Geometry: final body of the model. Coordinates: model frame, mm. Face numbers are marked on the shaded views. A direction names the side the tool comes from. Give positions to 0.01 mm unless a question says otherwise; leave off trailing zeros. Write each loop counter-clockwise with the first axis right and the second up, starting at its lowest first coordinate (ties: lowest second). Pieces come first, ordered by that corner, then holes. Notation, with made-up numbers: (25.25, -38) -> (30.25, -38) arc R18 ccw to (30.25, -22) -> close; hole circle Ø3 at (-39, -0.5). An arc over 180 degrees is marked (long way). Answer as a JSON object with one key per item and string values. Group by question number.
(1) Draft query along Y for the marked faces 4, 5 and 6. Return one class per face: +Y half, -Y half, draft (parallel to the pull), parting line (faces both ways), or undercut.
(2) Section query A-A on y = 15.5. Output: boundary loops of the cut face in (x, z), plus the area to 3 significant figures.
(3) Set-up query: the marked faces 1, 2 and 3. Return all of +Z, -Z, +X, -X, +Y, -Y with unobstructed straight access to the full face (end or side cutting, diameter ignored); none if empty.
(4) Contact query for flat-ended pins moving along their axis: pin 1 Ø12 at (y, z) = (25, 4) entering from +X; pin 2 Ø17 at (y, z) = (-0.5, -4.5) entering from +X; pin 3 Ø2 at (x, z) = (5.5, 12) entering from +Y; pin 4 Ø5 at (x, y) = (9.5, 3.5) entering from -Z. Output: stop coordinate, or through.
(5) Material intervals for probe 1 along Y at (x, z) = (4.25, 0); probe 2 along Y at (x, z) = (8.75, 0); probe 3 along X at (y, z) = (20.5, 13), sorted ascending.
(6) Section query C-C on y = -1. Output: boundary loops of the cut face in (x, z), plus the area to 3 significant figures.
(7) Section query B-B on x = 9. Output: boundary loops of the cut face in (y, z).
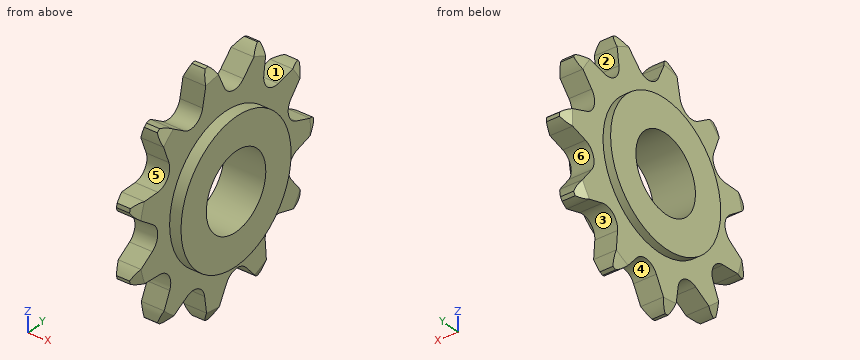
from build123d import *

# Parameters (mm, degrees)
SKETCH1_R           = 18.5
SKETCH1_R_2         = 10
BOSS_EXTRUDE1_DEPTH = 11
BOSS_EXTRUDE2_START = -6
SKETCH2_R           = 31.5
SKETCH2_R_2         = 10
BOSS_EXTRUDE2_DEPTH = 6
CHAMFER1_SIZE       = 1.27
CHAMFER1_SIZE2      = 2.723523789
CUT_EXTRUDE1_DEPTH  = 46.885727629
CIRPATTERN1_COUNT   = 11


with BuildPart() as part:
    # Sketch1 → Boss-Extrude1 (new body)
    with BuildSketch(Plane(origin=(0, 0, 0), x_dir=(0, 0, -1), z_dir=(1, 0, 0))):
        Circle(SKETCH1_R)
        Circle(SKETCH1_R_2, mode=Mode.SUBTRACT)
    extrude(amount=BOSS_EXTRUDE1_DEPTH)

    # Sketch2 → Boss-Extrude2 (add)
    with BuildSketch(Plane(origin=(7.999999904, 0, 0), x_dir=(0, 0, -1), z_dir=(1, 0, 0)).offset(BOSS_EXTRUDE2_START)):
        Circle(SKETCH2_R)
        Circle(SKETCH2_R_2, mode=Mode.SUBTRACT)
    extrude(amount=BOSS_EXTRUDE2_DEPTH)

    # Chamfer1
    chamfer1_edges = [part.edges().sort_by_distance(p)[0] for p in [
        (7.999999904, 0, 31.5),
        (1.999999904, 0, 31.5),
    ]]
    chamfer1_side = [part.faces().sort_by_distance(p)[0] for p in [
        (4.999999904, 0, 31.5),
    ]]
    chamfer(chamfer1_edges, length=CHAMFER1_SIZE, length2=CHAMFER1_SIZE2, reference=chamfer1_side[0])

    # Sketch3 → Cut-Extrude1 (cut, through all)
    with BuildSketch(Plane(origin=(11, 0, 0), x_dir=(0, 0, -1), z_dir=(1, 0, 0))):
        with BuildLine():
            Line((2.025004531, 28.705137864), (3.316836887, 24.373931538))
            ThreePointArc((3.316836887, 24.373931538), (5.909643301, 21.714368856), (9.571916138, 22.33378505))
            Line((9.571916138, 22.33378505), (13.570357606, 25.375795112))
            ThreePointArc((13.570357606, 25.375795112), (15.011752501, 26.239592723), (16.607426831, 26.766459872))
            ThreePointArc((16.607426831, 26.766459872), (16.819336008, 26.633811898), (17.03018575, 26.499486284))
            Line((17.03018575, 26.499486284), (18.753086107, 29.492558003))
            Line((18.753086107, 29.492558003), (0, 32.610896361))
            Line((0, 32.610896361), (0, 31.5))
            ThreePointArc((0, 31.5), (0.250007874, 31.499007858), (0.5, 31.496031496))
            ThreePointArc((0.5, 31.496031496), (1.409727709, 30.18103184), (2.025004531, 28.705137864))
        make_face()
    cut_extrude1 = extrude(amount=-CUT_EXTRUDE1_DEPTH, mode=Mode.SUBTRACT)

    # CirPattern1: Cut-Extrude1 ×11 about axis
    cirpattern1_axis = Axis((0, 0, 0), (1, 0, 0))
    for i in range(1, CIRPATTERN1_COUNT):
        add(cut_extrude1.rotate(cirpattern1_axis, i * 360 / CIRPATTERN1_COUNT), mode=Mode.SUBTRACT)


solid = part.part
Answer list:
{
 "1": {"face 4": "undercut", "face 5": "-Y half", "face 6": "+Y half"},
 "2": {"outline": "(0, -10.1) -> (2, -10.1) -> (2, -16.41) -> (8, -16.41) -> (8, -10.1) -> (11, -10.1) -> (11, 10.1) -> (8, 10.1) -> (8, 16.58) -> (2, 16.58) -> (2, 10.1) -> (0, 10.1) -> close", "area": "299 mm2"},
 "3": {"face 1": "+Z, +X, -X", "face 2": "+X, -X, +Y", "face 3": "+X, -X"},
 "4": {"pin 1": "x = 8", "pin 2": "x = 11", "pin 3": "y = 24.54", "pin 4": "z = -23.14"},
 "5": {"probe 1": "-22.51 to -10, 10 to 31.5", "probe 2": "-18.5 to -10, 10 to 18.5", "probe 3": "2 to 8"},
 "6": {"outline": "(0, -18.47) -> (2, -18.47) -> (2, -27.22) -> (8, -27.22) -> (8, -18.47) -> (11, -18.47) -> (11, -9.95) -> (0, -9.95) -> close; (0, 9.95) -> (11, 9.95) -> (11, 18.47) -> (8, 18.47) -> (8, 26.36) -> (2, 26.36) -> (2, 18.47) -> (0, 18.47) -> close", "area": "287 mm2"},
 "7": {"outline": "circle Ø37 at (0, 0); hole circle Ø20 at (0, 0)"}
}
